Geometry: final body of the model. Coordinates: model frame, mm. A direction names the side the tool comes from. Give positions to 0.01 mm unless a question says otherwise; leave off trailing zeros. Write each loop counter-clockwise with the first axis right and the second up, starting at its lowest first coordinate (ties: lowest second). Pieces come first, ordered by that corner, then holes.
Q1. Pin query (flat end, axial travel): pin 1 (2 mm diameter, centred on y = 15, z = -3.5, fed in from -X); pin 2 (1 mm diameter, centred on y = 20.5, z = 0, fed in from +X); pin 3 (2 mm diameter, centred on x = 0, y = 17.5, fed in from +Z). Return the tip coordinate at first contact, or that it passes through.
Q2. Cut plane D-D on y = 3.5. Return the cut outline in (x, z), plus the area to 3 significant figures.
Q3. Cut plane C-C on y = 16. Return the cut outline in (x, z).
Q4. Line query: L1, parallel to Y at x = -3.25, z = 0.5; L2, parallel to Y at x = -0.5, z = 2.75; L3, parallel to X at y = 13.5, z = 1.25. Output: solid intervals per line, ascending.
Q5. Reachability of faces 1 (the face through (-3.04, 31.97, 3.32)), 2 (the face through (3, 29.75, -1)) from +Z, -Z, +X, -X, +Y, -Y: full face, straight path, thin tool, end or side. Return the list, or none.
Q6. Cut plane A-A on x = 0. Return the cut outline in (y, z), plus the area to 3 significant figures.
Q7. Cut plane B-B on z = 0. Return the cut outline in (x, y), plus the area to 3 significant figures.
```python
from build123d import *


# Read off the part's stored shape, not the designer's step: M5 机械螺纹 螺柱1
with BuildPart() as part:
    # 草图1 → 旋转1 (revolve)
    with BuildSketch(Plane.XY, mode=Mode.PRIVATE) as revolve_1_sk:
        Polygon((0, 0), (0, 34.25), (4.5, 34.25), (4.5, 29.75), (3, 29.75), (3, 9.75), (2.8, 9.75), (2.8, 0), align=None)
    revolve(revolve_1_sk.sketch.rotate(Axis((0, 0, 0), (0, 1, 0)), 90), axis=Axis((0, 0, 0), (0, 1, 0)))

    # M5 机械螺纹 螺柱1 outline → M5 机械螺纹 螺柱1 (revolve, cut)
    with BuildSketch(Plane.XY):
        Polygon((2.8, 9.75), (2.5, 9.75), (2.5, 0.433), (2.067, 0), (2.8, 0), align=None)
    revolve(axis=Axis((0, 0, 0), (0, 1, 0)), mode=Mode.SUBTRACT)


solid = part.part
```
Data:
1. pin 1: stops at x = -1.66
1. pin 2: stops at x = 3
1. pin 3: stops at z = 3
2. outline: circle Ø5 at (0, 0)
2. area: 19.6 mm2
3. outline: circle Ø6 at (0, 0)
4. L1: y = 29.75 to 34.25
4. L2: y = 9.75 to 34.25
4. L3: x = -2.73 to 2.73
5. face 1: +Y, -Y
5. face 2: -Y
6. outline: (0, -2.07) - (0.43, -2.5) - (9.75, -2.5) - (9.75, -3) - (29.75, -3) - (29.75, -4.5) - (34.25, -4.5) - (34.25, 4.5) - (29.75, 4.5) - (29.75, 3) - (9.75, 3) - (9.75, 2.5) - (0.43, 2.5) - (0, 2.07) - close
6. area: 209 mm2
7. outline: (-4.5, 29.75) - (-3, 29.75) - (-3, 9.75) - (-2.5, 9.75) - (-2.5, 0.43) - (-2.07, 0) - (2.07, 0) - (2.5, 0.43) - (2.5, 9.75) - (3, 9.75) - (3, 29.75) - (4.5, 29.75) - (4.5, 34.25) - (-4.5, 34.25) - close
7. area: 209 mm2
